Can you work these out from the model? Positions are in its coordinate system, mm. A direction names the side the tool comes from. Round coordinates to 2 decimals unless told otherwise and drop trailing zeros. Order: outer loops, then holes, each group sorted by start corner. A loop starts at its lowest first (then second) coordinate and runs counter-clockwise, first axis right, second up.
from build123d import *

# Parameters (mm, degrees)
SKETCH1_W              = 177.8
SKETCH1_H              = 39.878
BOSS_EXTRUDE1_DEPTH    = 11.049
F_10_32_TAPPED_HOLE1_D = 4.0386
BOSS_EXTRUDE2_DEPTH    = 2.032


with BuildPart() as part:
    # Sketch1 → Boss-Extrude1 (new body)
    with BuildSketch(Plane(origin=(0, 0, 0), x_dir=(0, 0, -1), z_dir=(1, 0, 0))):
        Rectangle(SKETCH1_W, SKETCH1_H)
        with BuildLine():
            Line((-74.621306688, 6.6675), (74.621306688, 6.6675))
            ThreePointArc((74.621306688, 6.6675), (81.288806688, 0), (74.621306688, -6.6675))
            Line((74.621306688, -6.6675), (-74.621306688, -6.6675))
            ThreePointArc((-74.621306688, -6.6675), (-81.288806688, 0), (-74.621306688, 6.6675))
        make_face(mode=Mode.SUBTRACT)
    extrude(amount=BOSS_EXTRUDE1_DEPTH)

    # #10-32 Tapped Hole1 (through all)
    with Locations(Plane(origin=(11.049, 0, 0), x_dir=(0, 0, -1), z_dir=(1, 0, 0))):
        with Locations((-82.55, 13.589), (-82.55, -13.589), (0, -13.589), (82.55, -13.589), (82.55, 13.589), (0, 13.589)):
            Hole(F_10_32_TAPPED_HOLE1_D / 2)

    # Sketch5 → Boss-Extrude2 (add)
    with BuildSketch(Plane.ZY):
        with BuildLine():
            Line((-36.521306688, -6.6675), (74.621306688, -6.6675))
            ThreePointArc((74.621306688, -6.6675), (81.288806688, 0), (74.621306688, 6.6675))
            Line((74.621306688, 6.6675), (-36.521306688, 6.6675))
            ThreePointArc((-36.521306688, 6.6675), (-29.853806688, 0), (-36.521306688, -6.6675))
        make_face()
    extrude(amount=-BOSS_EXTRUDE2_DEPTH)


solid = part.part
(1) I want a section at A-A, the plane y = 0. List the corners of the cut face in (x, z) for me, plus the area to 3 significant figures.
(2) I want a section at D-D, the plane z = -25. List the corners of the cut face in (x, y) for me.
(3) I want a section at C-C, the plane x = 5.75. Give the number of separate pieces and of enclosed holes in the cut face, plus the area to 3 significant figures.
(4) I'm going to push flat-ended pins straight in: pin 1 Ø2 at (y, z) = (6, -65) entering from -X; pin 2 Ø4 at (y, z) = (0.5, 18) entering from +X. Where does each tip first touch, or does it pass through?
(5) On a 3-axis mill with a long thin cutter (end or side, diameter ignored), from which of +Z, -Z, +X, -X, +Y, -Y can I reach the whole of each face in a straight line? I mean faces 4 (the face through (6.477, -0.147, 81.287)), 5 (the face through (11.049, 9, 1)), 6 (the face through (5.447, 0.147, -81.287)). Say none if no direction works.
(6) If we mould it in two halves opening along Y, with no side actions, what happens to faces 1 (the face through (5, -19.939, 1)), 2 (the face through (0, 0, -1)), 3 (the face through (1.002, 0.147, -29.855))? For each: pulls with the +Y half, pulls with the -Y half, needs draft (parallel to the pull), parting line crosses it, or undercut.
(7) Please list where these lines run through material, in increasing order: probe 1 along Y at (x, z) = (6.25, 0); probe 2 along Y at (x, z) = (5.25, -82.55); probe 3 along Y at (x, z) = (4, 35).
(8) I want a section at B-B, the plane z = 0. List the corners of the cut face in (x, y) for me, plus the area to 3 significant figures.
Ans:
1. outline: (0, -88.9) - (11.05, -88.9) - (11.05, -81.29) - (0, -81.29) - close; (0, -29.85) - (2.03, -29.85) - (2.03, 81.29) - (11.05, 81.29) - (11.05, 88.9) - (0, 88.9) - close
1. area: 394 mm2
2. outline: (0, -19.94) - (11.05, -19.94) - (11.05, -6.67) - (2.03, -6.67) - (2.03, 6.67) - (11.05, 6.67) - (11.05, 19.94) - (0, 19.94) - close
3. separate pieces: 1
3. enclosed holes: 7
3. area: 4,880 mm2
4. pin 1: stops at x = 0
4. pin 2: stops at x = 2.03
5. face 4: +X
5. face 5: +Z, -Z, +X, +Y, -Y
5. face 6: +X, -X
6. face 1: pulls with the -Y half
6. face 2: needs draft
6. face 3: undercut
7. probe 1: y = -19.94 to -15.61, -11.57 to -6.67, 6.67 to 11.57, 15.61 to 19.94
7. probe 2: y = -19.94 to -15.61, -11.57 to 11.57, 15.61 to 19.94
7. probe 3: y = -19.94 to -6.67, 6.67 to 19.94
8. outline: (0, -19.94) - (11.05, -19.94) - (11.05, -15.61) - (0, -15.61) - close; (0, -11.57) - (11.05, -11.57) - (11.05, -6.67) - (2.03, -6.67) - (2.03, 6.67) - (11.05, 6.67) - (11.05, 11.57) - (0, 11.57) - close; (0, 15.61) - (11.05, 15.61) - (11.05, 19.94) - (0, 19.94) - close
8. area: 231 mm2
